Here's how the part is built. I have some questions about the finished solid (model axes, mm). Face numbers are marked on the shaded views. A direction names the side the tool comes from. Round coordinates to 2 decimals unless told otherwise and drop trailing zeros. Loops run counter-clockwise (first coordinate to the right, second up) from the corner with the lowest first, then second, coordinate; pieces in that order, holes last. Notation, with made-up numbers: (73, 75) - (112, 75) arc R29 ccw to (112, 96) - close; hole circle Ø11 at (44, 23). An arc over 180 degrees is marked (long way). Answer as a JSON object with one key per item and string values. Group by question number.
1) I want a section at B-B, the plane x = -3.5. Please give me the cut outline in (y, z).
2) Will these pins go through, and if not, where does the flat tip stop? P1, Ø4, axis at x = 3, y = -14.5, coming from the +Z side; P2, Ø12, axis at x = 12.5, y = 5, coming from the +Z side; P3, Ø3, axis at y = -14.5, z = 4.5, coming from the +X side.
3) I want a section at A-A, the plane z = 3.75. Please give me the cut outline in (x, y).
4) If I drill on line 1 along Z through (x, y) = (7.5, -38.9); line 2 along Y through (x, z) = (4.5, 2.25); line 3 along Y through (x, z) = (3.5, 16), over which ranges is the centre line in solid material (lowest first)? Write a range as [from, to].
5) Which directions (+Z, -Z, +X, -X, +Y, -Y) give clear straight access to the entire face, cutting with the end or side of a thin tool? Please do the marked faces 1, 2 and 3.
6) I want a section at C-C, the plane z = 10. Please give me the cut outline in (x, y), then the cut area to 3 significant figures.
7) I want a section at D-D, the plane x = 0. Please give me the cut outline in (y, z), then the cut area to 3 significant figures.
8) If we mould it in two halves opening along X, with no side actions, what happens to the marked faces 4, 5 and 6? For each: pulls with the +X half, pulls with the -X half, needs draft (parallel to the pull), parting line crosses it, or undercut.
from build123d import *

# Parameters (mm, degrees)
F0_W      = 32.16
F0_H      = 31
F1_DEPTH  = 2
F3_D      = 2.1
F3_DEPTH  = 5
F3_TIP    = 0.63090365
F4_W      = 16.8
F4_H      = 2.5
F5_DEPTH  = 6.5
F6_DEPTH  = 25
F7_W      = 16.8
F7_H      = 23.7160715014
F8_DEPTH  = 25
F9_W      = 6.8209058344
F9_H      = 2
F10_DEPTH = 18
F11_W     = 32.16
F11_H     = 2.5
F12_DEPTH = 22
F14_D     = 3.4
F14_DEPTH = 5
F14_TIP   = 1.0214630523
F15_DEPTH = 0.2
F16_DEPTH = 0.2
F17_R     = 5


with BuildPart() as f1:
    # F0 (on Top) → F1 (new body)
    with BuildSketch(Plane.XY):
        Rectangle(F0_W, F0_H)
    extrude(amount=F1_DEPTH)

    # F3
    with Locations(Plane.XY.offset(2)):
        with Locations((-14.1555870968, 13.645), (14.1555870968, 13.645), (-14.1555870968, -13.645), (14.1555870968, -13.645)):
            Hole(F3_D / 2, depth=F3_DEPTH)
            with Locations((0, 0, -(F3_DEPTH + F3_TIP / 2))):  # 118° drill point
                Cone(0, F3_D / 2, F3_TIP, mode=Mode.SUBTRACT)

    # F4 (on face) → F5 (join)
    with BuildSketch(Plane.XY.offset(2)):
        with Locations((0, -14.25)):
            Rectangle(F4_W, F4_H)
    extrude(amount=F5_DEPTH)

    # F6 (add): a face of the model
    f6_faces = [f1.faces().sort_by_distance(p)[0] for p in [
        (0, -15.5, 3.6746196404),
    ]]
    extrude(f6_faces, amount=F6_DEPTH)

    # F7 (on face) → F8 (cut)
    with BuildSketch(Plane.XY.offset(8.5)):
        with Locations((0, -28.6419642493)):
            Rectangle(F7_W, F7_H)
    extrude(amount=-F8_DEPTH, mode=Mode.SUBTRACT)

    # F9 (on face) → F10 (join)
    with BuildSketch(Plane(origin=(8.4, 0, 0), x_dir=(0, -1, 0), z_dir=(-1, 0, 0))):
        with Locations((37.0895470828, 1)):
            Rectangle(F9_W, F9_H)
    extrude(amount=F10_DEPTH)

    # F11 (on face) → F12 (join)
    with BuildSketch(Plane(origin=(0, 0, 0), x_dir=(1, 0, 0), z_dir=(0, 0, -1))):
        with Locations((0, 39.25)):
            Rectangle(F11_W, F11_H)
    extrude(amount=-F12_DEPTH)

    # F14
    with Locations(Plane.XZ.offset(40.5)):
        with Locations((-7.5, 17.5), (-7.5, 10), (0, 10), (0, 17.5), (7.5, 17.5), (7.5482047356, 10)):
            Hole(F14_D / 2, depth=F14_DEPTH)
            with Locations((0, 0, -(F14_DEPTH + F14_TIP / 2))):  # 118° drill point
                Cone(0, F14_D / 2, F14_TIP, mode=Mode.SUBTRACT)

    # F15 (cut): a face of the model
    f15_faces = [f1.faces().sort_by_distance(p)[0] for p in [
        (8.4, -14.8919642493, 5.25),
    ]]
    extrude(f15_faces, amount=-F15_DEPTH, mode=Mode.SUBTRACT)

    # F16 (cut): a face of the model
    f16_faces = [f1.faces().sort_by_distance(p)[0] for p in [
        (-8.4, -14.8919642493, 5.25),
    ]]
    extrude(f16_faces, amount=-F16_DEPTH, mode=Mode.SUBTRACT)

    # F17
    f17_edges = [f1.edges().sort_by_distance(p)[0] for p in [
        (-16.08, -39.25, 22),
        (16.08, -39.25, 22),
    ]]
    fillet(f17_edges, radius=F17_R)


solid = f1.part
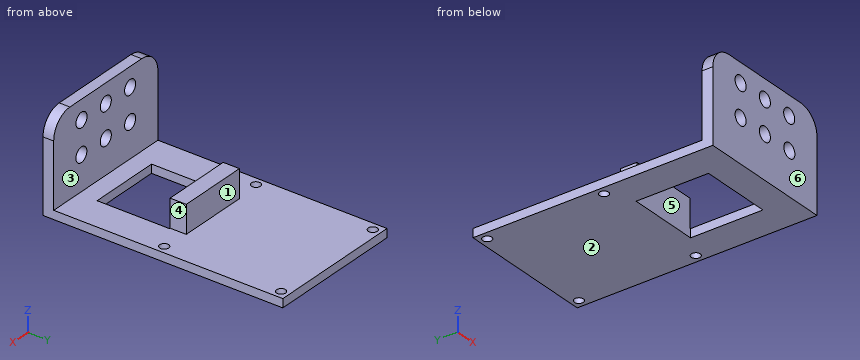
Outcome:
{
 "1": {"outline": "(-40.5, 0) - (-33.68, 0) - (-33.68, 2) - (-38, 2) - (-38, 22) - (-40.5, 22) - close; (-16.78, 0) - (15.5, 0) - (15.5, 2) - (-13, 2) - (-13, 8.5) - (-16.78, 8.5) - close"},
 "2": {"P1": "z = 8.5", "P2": "z = 2", "P3": "x = 8.2"},
 "3": {"outline": "(-16.08, -40.5) - (16.08, -40.5) - (16.08, -38) - (-16.08, -38) - close; (-8.2, -16.78) - (8.2, -16.78) - (8.2, -13) - (-8.2, -13) - close"},
 "4": {"line 1": "[0, 8.3], [11.7, 15.8], [19.2, 22]", "line 2": "[-40.5, -38], [-16.78, -13]", "line 3": "[-40.5, -38]"},
 "5": {"face 1": "+Z, +X, -X, +Y", "face 2": "-Z, +X, -X, +Y, -Y", "face 3": "+Z, +X, -X"},
 "6": {"outline": "(-16.08, -40.5) - (-9.2, -40.5) - (-9.2, -38) - (-16.08, -38) - close; (-5.8, -40.5) - (-1.7, -40.5) - (-1.7, -38) - (-5.8, -38) - close; (1.7, -40.5) - (5.85, -40.5) - (5.85, -38) - (1.7, -38) - close; (9.25, -40.5) - (16.08, -40.5) - (16.08, -38) - (9.25, -38) - close", "area": "54.9 mm^2"},
 "7": {"outline": "(-40.5, 0) - (-33.68, 0) - (-33.68, 2) - (-38, 2) - (-38, 8.3) - (-40.5, 8.3) - close; (-40.5, 11.7) - (-38, 11.7) - (-38, 15.8) - (-40.5, 15.8) - close; (-40.5, 19.2) - (-38, 19.2) - (-38, 22) - (-40.5, 22) - close; (-16.78, 0) - (15.5, 0) - (15.5, 2) - (-13, 2) - (-13, 8.5) - (-16.78, 8.5) - close", "area": "136 mm^2"},
 "8": {"face 4": "pulls with the +X half", "face 5": "undercut", "face 6": "needs draft"}
}
